Here's how the part is built. I have some questions about the finished solid (model axes, mm). Face numbers are marked on the shaded views. A direction names the side the tool comes from. Round coordinates to 2 decimals unless told otherwise and drop trailing zeros. Loops run counter-clockwise (first coordinate to the right, second up) from the corner with the lowest first, then second, coordinate; pieces in that order, holes last. Notation, with made-up numbers: (84.25, 61.5) - (95.25, 61.5) arc R26 ccw to (95.25, 77.5) - close; hole circle Ø4 at (-8, 81.5). An arc over 180 degrees is marked (long way). Answer as a JSON object with one key per item and string values. Group by question number.
1) Which directions (+Z, -Z, +X, -X, +Y, -Y) give clear straight access to the entire face, cutting with the end or side of a thin tool? Please do the marked faces 4, 5, 6 and 7.
2) Will these pins go through, and if not, where does the flat tip stop? P1, Ø11.5, axis at x = -17, z = -20.5, coming from the -Y side; P2, Ø2.5, axis at x = -10.5, z = -10.5, coming from the +Y side; P3, Ø3, axis at x = 0, z = 20, coming from the -Y side.
3) If we mould it in two halves opening along X, with no side actions, what happens to the marked faces 1, 2 and 3? For each: pulls with the +X half, pulls with the -X half, needs draft (parallel to the pull), parting line crosses it, or undercut.
4) I want a section at A-A, the plane z = -10. Please give me the cut outline in (x, y), then the cut area to 3 significant figures.
5) If I drill on line 1 along X through (y, z) = (3.9, 10); line 2 along X through (y, z) = (-1.25, 0), over which ranges is the centre line in solid material (lowest first)? Write a range as [from, to].
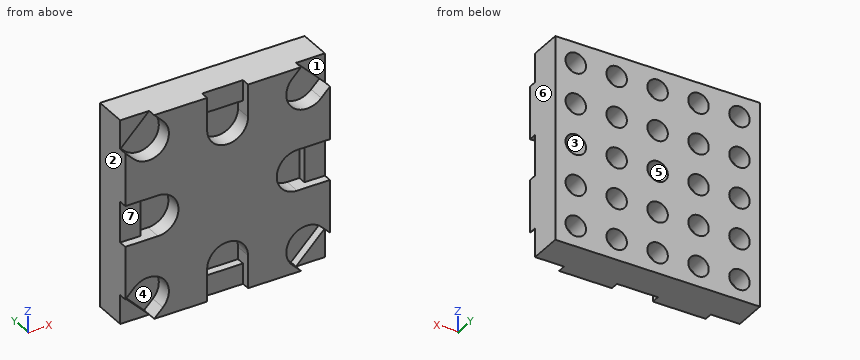
Autodesk Inventor part; units mm, degrees
sketch "Sketch1" plane through (0, 0, 0) normal (0, 1, 0) x (-1, 0, 0)
  line L0 (25, -25) -> (-25, -25)
  line L1 (-25, -25) -> (-25, 25)
  line L2 (-25, 25) -> (25, 25)
  line L3 (25, 25) -> (25, -25)
  line L4 (0, -35) -> (0, 35)
  line L5 (-35, 0) -> (35, 0)
  point P0 (0, 0)
  point P1 (0, -25)
  point P2 (25, 0)
  dimension "d0" = 50
  dimension "d1" = 50
extrude "Extrusion1" add sketch "Sketch1" along normal mid plane 10
sketch "Sketch2" plane through (0, -5, 0) normal (0, -1, 0) x (1, 0, 0)
  line L0 (-25, -25) -> (-25, 25)
  line L1 (-25, 5) -> (-17, 5)
  line L2 (-17, 5) -> (-17, -5)
  line L3 (-17, -5) -> (-25, -5)
  line L4 (-25, -5) -> (-25, 5)
  arc A0 (-17, -5) -> (-17, 5) centre (-17, 0) ccw
  line L5 (-35, 0) -> (35, 0)
  line L6 (-20, 5) -> (-20, -5)
  line L7 (0, -35) -> (0, 35)
  line L8 (-5, -25) -> (-5, -17)
  arc A1 (5, -17) -> (-5, -17) centre (0, -17) ccw
  line L9 (5, -17) -> (5, -25)
  line L10 (5, -25) -> (-5, -25)
  line L11 (-5, -20) -> (5, -20)
  line L12 (-5, -17) -> (5, -17)
  line L13 (25, -5) -> (17, -5)
  arc A2 (17, 5) -> (17, -5) centre (17, 0) ccw
  line L14 (17, 5) -> (25, 5)
  line L15 (25, 5) -> (25, -5)
  line L16 (20, -5) -> (20, 5)
  line L17 (17, -5) -> (17, 5)
  line L18 (5, 25) -> (5, 17)
  arc A3 (-5, 17) -> (5, 17) centre (0, 17) ccw
  line L19 (-5, 17) -> (-5, 25)
  line L20 (-5, 25) -> (5, 25)
  line L21 (5, 20) -> (-5, 20)
  line L22 (5, 17) -> (-5, 17)
  line L23 (25, -25) -> (19.3431, -19.3431)
  line L24 (15.8076, -22.8787) -> (22.8787, -15.8076)
  line L25 (25, -25) -> (-25, -25)
  line L26 (17.9289, -25) -> (25, -25)
  line L27 (25, -25) -> (25, -17.9289)
  line L28 (25, 25) -> (25, -25)
  line L29 (17.9289, -25) -> (15.8076, -22.8787)
  line L30 (25, -17.9289) -> (22.8787, -15.8076)
  line L31 (17.9289, -25) -> (25, -17.9289)
  arc A4 (22.8787, -15.8076) -> (15.8076, -22.8787) centre (19.3431, -19.3431) ccw
  line L32 (25, 17.9289) -> (22.8787, 15.8076)
  arc A5 (15.8076, 22.8787) -> (22.8787, 15.8076) centre (19.3431, 19.3431) ccw
  line L33 (22.8787, 15.8076) -> (15.8076, 22.8787)
  line L34 (17.9289, 25) -> (15.8076, 22.8787)
  line L35 (25, 17.9289) -> (17.9289, 25)
  line L36 (25, 17.9289) -> (25, 25)
  line L37 (25, 25) -> (19.3431, 19.3431)
  line L38 (25, 25) -> (17.9289, 25)
  line L39 (-17.9289, 25) -> (-15.8076, 22.8787)
  arc A6 (-22.8787, 15.8076) -> (-15.8076, 22.8787) centre (-19.3431, 19.3431) ccw
  line L40 (-15.8076, 22.8787) -> (-22.8787, 15.8076)
  line L41 (-25, 17.9289) -> (-22.8787, 15.8076)
  line L42 (-17.9289, 25) -> (-25, 17.9289)
  line L43 (-17.9289, 25) -> (-25, 25)
  line L44 (-25, 25) -> (-19.3431, 19.3431)
  line L45 (-25, 25) -> (-25, 17.9289)
  line L46 (-25, -17.9289) -> (-22.8787, -15.8076)
  arc A7 (-15.8076, -22.8787) -> (-22.8787, -15.8076) centre (-19.3431, -19.3431) ccw
  line L47 (-22.8787, -15.8076) -> (-15.8076, -22.8787)
  line L48 (-17.9289, -25) -> (-15.8076, -22.8787)
  line L49 (-25, -17.9289) -> (-17.9289, -25)
  line L50 (-25, -17.9289) -> (-25, -25)
  line L51 (-25, -25) -> (-19.3431, -19.3431)
  line L52 (-25, -25) -> (-17.9289, -25)
  point P0 (0, 0)
  point P1 (-25, 0)
  point P2 (0, -25)
  point P3 (25, 0)
  point P4 (0, 25)
  dimension "d4" = 10
  dimension "d5" = 8
  dimension "d6" = 3
  dimension "d9" = 360
  dimension "d28" = 8
  dimension "d31" = 3
  dimension "d33" = 135
  dimension "d34" = 3
  dimension "d35" = 10
  dimension "d36" = 45
  dimension "d39" = 360
extrude "Extrusion2" cut sketch "Sketch2" against normal blind 2 contours L0 L44 L42 | L35 L37 L28 | L51 L49 L25 | L0 L49 L51 | L0 L5 L6 L3 | L8 L11 L7 L10 | L0 L1 L6 L5 | L7 L11 L9 L10 | L31 L23 L25 | L43 L42 L44 | L23 L31 L27 | L13 L16 L5 L15 | L16 L14 L15 L5 | L21 L19 L20 L7 | L7 L20 L18 L21 | L37 L35 L38
extrude "Extrusion3" cut sketch "Sketch2" against normal blind 4 contours L42 L44 L40 L41 | A3 L22 L7 | L7 L22 A3 | L32 L33 L37 L35 | L46 L47 L51 L49 | L49 L51 L47 L48 | A7 L47 | L6 L5 L2 L3 | L8 L12 L7 L11 | L6 L1 L2 L5 | L2 L5 A0 | A1 L7 L12 | L7 L12 L9 L11 | L2 A0 L5 | A1 L12 L7 | L29 L24 L23 L31 | L40 A6 | L42 L39 L40 L44 | A4 L24 | L23 L24 L30 L31 | A2 L17 L5 | L5 L17 A2 | L17 L14 L16 L5 | L5 L16 L13 L17 | L22 L19 L21 L7 | L7 L21 L18 L22 | A5 L33 | L37 L33 L34 L35
sketch "Sketch3" plane through (0, 5, 0) normal (0, 1, 0) x (1, 0, 0)
  circle A0 centre (-20, 20) radius 2.5
  line L0 (25, 25) -> (-25, 25)
  line L1 (-25, 25) -> (-25, -25)
  line L2 (-35, 0) -> (35, 0)
  line L3 (0, 35) -> (0, -35)
  circle A1 centre (-20, 10) radius 2.5
  circle A2 centre (-20, 0) radius 2.5
  circle A3 centre (-20, -10) radius 2.5
  circle A4 centre (-20, -20) radius 2.5
  circle A5 centre (-10, 20) radius 2.5
  circle A6 centre (-10, 10) radius 2.5
  circle A7 centre (-10, 0) radius 2.5
  circle A8 centre (-10, -10) radius 2.5
  circle A9 centre (-10, -20) radius 2.5
  circle A10 centre (0, 20) radius 2.5
  circle A11 centre (0, 10) radius 2.5
  circle A12 centre (0, 0) radius 2.5
  circle A13 centre (0, -10) radius 2.5
  circle A14 centre (0, -20) radius 2.5
  circle A15 centre (10, 20) radius 2.5
  circle A16 centre (10, 10) radius 2.5
  circle A17 centre (10, 0) radius 2.5
  circle A18 centre (10, -10) radius 2.5
  circle A19 centre (10, -20) radius 2.5
  circle A20 centre (20, 20) radius 2.5
  circle A21 centre (20, 10) radius 2.5
  circle A22 centre (20, 0) radius 2.5
  circle A23 centre (20, -10) radius 2.5
  circle A24 centre (20, -20) radius 2.5
  dimension "d15" = 5
  dimension "d16" = 5
  dimension "d17" = 5
  dimension "d20" = 10
  dimension "d23" = 10
extrude "Extrusion4" cut sketch "Sketch3" against normal blind 5 contours A0 | A22 L2 | L2 A22 | A17 L2 | L2 A17 | A14 L3 | L3 A14 | A13 L3 | L3 A13 | A10 L3 | L3 A10 | A2 L2 | L2 A2 | A11 L3 | L3 A11 | A7 L2 | L2 A7 | A12 L2 L3 | L3 L2 A12 | L3 A12 L2 | L2 A12 L3 | A1 | A3 | A4 | A5 | A6 | A8 | A9 | A15 | A16 | A18 | A19 | A20 | A21 | A23 | A24
properties part number "Tile"
Outcome:
{
 "1": {"face 4": "-Y", "face 5": "+Y", "face 6": "+Z, -Z, +X, +Y, -Y", "face 7": "-X, -Y"},
 "2": {"P1": "y = -5", "P2": "y = 0", "P3": "y = -3"},
 "3": {"face 1": "needs draft", "face 2": "pulls with the -X half", "face 3": "undercut"},
 "4": {"outline": "(-25, -5) - (25, -5) - (25, 5) - (22.5, 5) - (22.5, 0) - (17.5, 0) - (17.5, 5) - (12.5, 5) - (12.5, 0) - (7.5, 0) - (7.5, 5) - (2.5, 5) - (2.5, 0) - (-2.5, 0) - (-2.5, 5) - (-7.5, 5) - (-7.5, 0) - (-12.5, 0) - (-12.5, 5) - (-17.5, 5) - (-17.5, 0) - (-22.5, 0) - (-22.5, 5) - (-25, 5) - close", "area": "375 mm^2"},
 "5": {"line 1": "[-25, -22.5], [-17.5, -12.5], [-7.5, -2.5], [2.5, 7.5], [12.5, 17.5], [22.5, 25]", "line 2": "[-25, -20], [-12, 12], [20, 25]"}
}
